from build123d import *

# Parameters (mm, degrees)
F0_W        = 78
F0_H        = 15
F1_DEPTH    = 109
F2_T        = -2
F4_DEPTH    = 109
F6_DEPTH    = 78
F7_T1_DEPTH = 23


# Not quite as in the source:
# - a fillet or chamfer that OpenCascade refuses, or shapes differently, is made with other operations: its cross-section is extruded or revolved along the edge and cut away or added


with BuildPart() as f1:
    # F0 (on Front) → F1 (new body)
    with BuildSketch(Plane.XZ):
        with Locations((39, -7.5)):
            Rectangle(F0_W, F0_H)
    extrude(amount=-F1_DEPTH)

    # F2
    f2_openings = [f1.faces().sort_by_distance(p)[0] for p in [
        (39, 54.5, 0),
    ]]
    offset(amount=F2_T, openings=f2_openings)

    # F3 (on face) → F4 (join, through all)
    with BuildSketch(Plane.XZ):
        Polygon((0, 2), (0, 0), (1.2, 0), (2, 1), (2, 2), align=None)
        Polygon((76, 1), (76.8, 0), (78, 0), (78, 2), (76, 2), align=None)
    extrude(amount=-F4_DEPTH)

    # F5 (on face) → F6 (join, through all)
    with BuildSketch(Plane.YZ.offset(78)):
        Polygon((109, 0), (109, 2), (107, 2), (107, 1), (107.8, 0), align=None)
    extrude(amount=-F6_DEPTH)

    # F7: fillet of radius 1.2 on 4 edges, made by hand

    # F7_s2 → F7_t1 (cut)
    with BuildSketch(Plane.XY.offset(-18)):
        with BuildLine():
            add(Edge.make_bspline(
                [(78, 1.2), (78, 0), (76.8, 0)],
                knots=[0, 0, 0, 1, 1, 1], degree=2, weights=[1, 1, 1]))
            Line((76.8, 0), (78, 0))
            Line((78, 0), (78, 1.2))
        make_face()
        with BuildLine():
            add(Edge.make_bspline(
                [(76.8, 109), (78, 109), (78, 107.8)],
                knots=[0, 0, 0, 1, 1, 1], degree=2, weights=[1, 1, 1]))
            Line((78, 107.8), (78, 109))
            Line((78, 109), (76.8, 109))
        make_face()
        with BuildLine():
            add(Edge.make_bspline(
                [(0, 107.8), (0, 109), (1.2, 109)],
                knots=[0, 0, 0, 1, 1, 1], degree=2, weights=[1, 1, 1]))
            Line((1.2, 109), (0, 109))
            Line((0, 109), (0, 107.8))
        make_face()
        with BuildLine():
            add(Edge.make_bspline(
                [(0, 1.2), (0, 0), (1.2, 0)],
                knots=[0, 0, 0, 1, 1, 1], degree=2, weights=[1, 1, 1]))
            Line((1.2, 0), (0, 0))
            Line((0, 0), (0, 1.2))
        make_face()
    extrude(amount=F7_T1_DEPTH, mode=Mode.SUBTRACT)


solid = f1.part
CAD build for the part. Positions are in the model's coordinates, mm. A direction names the side the tool comes from. Coordinates: 2 decimals unless noted, no trailing zeros. Loops run counter-clockwise (first coordinate to the right, second up) from the corner with the lowest first, then second, coordinate; pieces in that order, holes last. Notation, with made-up numbers: (-4.75, 85) - (21.25, 85) arc R26 cw to (21.25, 99) - close; hole circle Ø10 at (60, 18). An arc over 180 degrees is marked (long way). Write item = value, one per line. Start each with the question number.
Q1. Cut at A-A, the plane x = 43. List the corners of the cut face in (y, z), then the cut area to 3 significant figures.
Q2. Pull direction Y, two halves, no side cores. Call faces 1 (the flat face through (38, 0, -7)), 2 (the flat face through (38, 2, -6)), 3 (the flat face through (38, 107, -6)), 4 (the flat face through (77, 54, 2)): pulls with the +Y half, pulls with the -Y half, needs draft (parallel to the pull), parting line crosses it, or undercut.
Q3. Drill centre lines: L1, parallel to Y at x = 18, z = -3.75; L2, parallel to X at y = 11.5, z = -11.25; L3, parallel to Z at x = 7, y = 46.5. Where is each one in solid material? Low to high.
Q4. Which spindle directions (+Z, -Z, +X, -X, +Y, -Y) get a long thin tool onto all of the face, cutting with end or side? Do faces 5 (the flat face through (78, 54, -7)), 6 (the flat face through (2, 54, -7)). Say none if no direction does.
Q5. Cut at B-B, the plane y = 29. List the corners of the cut face in (x, z).
Q6. Flat gauge pins, fed straight in: pin 1 Ø8 at (x, y) = (52.5, 93) entering from +Z; pin 2 Ø0.5 at (x, z) = (38, 1.5) entering from -Y. Where does each tip first touch, or does it go through?
Computed:
q1.outline = (0, -15) - (109, -15) - (109, 2) - (107, 2) - (107, 1) - (107.8, 0) - (107, 0) - (107, -13) - (2, -13) - (2, 0) - (0, 0) - close
q1.area = 274 mm²
q2.face_1 = pulls with the -Y half
q2.face_2 = undercut
q2.face_3 = undercut
q2.face_4 = needs draft
q3.L1 = 0 to 2, 107 to 109
q3.L2 = 0 to 2, 76 to 78
q3.L3 = -15 to -13
q4.face_5 = +Z, -Z, +X, +Y, -Y
q4.face_6 = +Z
q5.outline = (0, -15) - (78, -15) - (78, 2) - (76, 2) - (76, 1) - (76.8, 0) - (76, 0) - (76, -13) - (2, -13) - (2, 0) - (1.2, 0) - (2, 1) - (2, 2) - (0, 2) - close
q6.pin_1 = -13
q6.pin_2 = 107
